```python
from build123d import *

# Parameters (mm, degrees)
ESQUISSE1_W                          = 6
ESQUISSE1_H                          = 3.2
EXTRUSION1_DEPTH                     = 22.64
ENL_V_MAT_EXTRU_1_DEPTH              = 0.5
ESQUISSE3_R                          = 0.25
R_P_TITION_LIN_AIRE1_COUNT           = 9
R_P_TITION_LIN_AIRE1_PITCH           = 2.54
R_P_TITION_LIN_AIRE1_COPY_1_SKETCH_R = 0.25
R_P_TITION_LIN_AIRE1_COPY_2_SKETCH_R = 0.25
R_P_TITION_LIN_AIRE1_COPY_3_SKETCH_R = 0.25
R_P_TITION_LIN_AIRE1_COPY_4_SKETCH_R = 0.25
R_P_TITION_LIN_AIRE1_COPY_5_SKETCH_R = 0.25
R_P_TITION_LIN_AIRE1_COPY_6_SKETCH_R = 0.25
R_P_TITION_LIN_AIRE1_COPY_7_SKETCH_R = 0.25
R_P_TITION_LIN_AIRE1_COPY_8_SKETCH_R = 0.25


with BuildPart() as part:
    # Esquisse1 → Extrusion1 (new body)
    with BuildSketch(Plane(origin=(0, 0, 0), x_dir=(0, 0, -1), z_dir=(1, 0, 0))):
        with Locations((0, 1.6)):
            Rectangle(ESQUISSE1_W, ESQUISSE1_H)
    extrude(amount=EXTRUSION1_DEPTH)

    # Esquisse2 → Enlèv. mat.-Extru.1 (cut)
    with BuildSketch(Plane(origin=(0, 3.2, 0), x_dir=(-1, 0, 0), z_dir=(0, 1, 0))):
        with BuildLine():
            Line((0, -1), (0, 1))
            ThreePointArc((0, 1), (-1, 0), (0, -1))
        make_face()
    extrude(amount=-ENL_V_MAT_EXTRU_1_DEPTH, mode=Mode.SUBTRACT)

    # Balayage1: sweep along a path in Esquisse5
    with BuildLine(Plane(origin=(1.16, 0, 0), x_dir=(0, 0, -1), z_dir=(1, 0, 0))) as balayage1_path:
        Line((-3, 1.6), (-3.65, 1.6))
        Line((-3.65, 1.6), (-3.65, -4))
    # Esquisse3 → Balayage1 (sweep)
    with BuildSketch(Plane.XY.offset(3)):
        with Locations((1.16, 1.6)):
            Circle(ESQUISSE3_R)
    balayage1 = sweep(path=balayage1_path.line, transition=Transition.RIGHT)

    # Symétrie1: Balayage1 across plane
    add(balayage1.mirror(Plane.XY))

    # Répétition linéaire1: Balayage1 ×9
    with Locations(*[(i * R_P_TITION_LIN_AIRE1_PITCH, 0, 0) for i in range(1, R_P_TITION_LIN_AIRE1_COUNT)]):
        add(balayage1)

    # Répétition linéaire1 copy 1: sweep along a path in Répétition linéaire1 copy 1 path
    with BuildLine(Plane(origin=(3.7, 0, 0), x_dir=(0, 0, 1), z_dir=(1, 0, 0))) as r_p_tition_lin_aire1_copy_1_path:
        Line((-3, -1.6), (-3.65, -1.6))
        Line((-3.65, -1.6), (-3.65, 4))
    # Répétition linéaire1 copy 1 sketch → Répétition linéaire1 copy 1 (sweep)
    with BuildSketch(Plane(origin=(2.54, 0, -3), x_dir=(1, 0, 0), z_dir=(0, 0, -1))):
        with Locations((1.16, -1.6)):
            Circle(R_P_TITION_LIN_AIRE1_COPY_1_SKETCH_R)
    sweep(path=r_p_tition_lin_aire1_copy_1_path.line, transition=Transition.RIGHT)

    # Répétition linéaire1 copy 2: sweep along a path in Répétition linéaire1 copy 2 path
    with BuildLine(Plane(origin=(6.24, 0, 0), x_dir=(0, 0, 1), z_dir=(1, 0, 0))) as r_p_tition_lin_aire1_copy_2_path:
        Line((-3, -1.6), (-3.65, -1.6))
        Line((-3.65, -1.6), (-3.65, 4))
    # Répétition linéaire1 copy 2 sketch → Répétition linéaire1 copy 2 (sweep)
    with BuildSketch(Plane(origin=(5.08, 0, -3), x_dir=(1, 0, 0), z_dir=(0, 0, -1))):
        with Locations((1.16, -1.6)):
            Circle(R_P_TITION_LIN_AIRE1_COPY_2_SKETCH_R)
    sweep(path=r_p_tition_lin_aire1_copy_2_path.line, transition=Transition.RIGHT)

    # Répétition linéaire1 copy 3: sweep along a path in Répétition linéaire1 copy 3 path
    with BuildLine(Plane(origin=(8.78, 0, 0), x_dir=(0, 0, 1), z_dir=(1, 0, 0))) as r_p_tition_lin_aire1_copy_3_path:
        Line((-3, -1.6), (-3.65, -1.6))
        Line((-3.65, -1.6), (-3.65, 4))
    # Répétition linéaire1 copy 3 sketch → Répétition linéaire1 copy 3 (sweep)
    with BuildSketch(Plane(origin=(7.62, 0, -3), x_dir=(1, 0, 0), z_dir=(0, 0, -1))):
        with Locations((1.16, -1.6)):
            Circle(R_P_TITION_LIN_AIRE1_COPY_3_SKETCH_R)
    sweep(path=r_p_tition_lin_aire1_copy_3_path.line, transition=Transition.RIGHT)

    # Répétition linéaire1 copy 4: sweep along a path in Répétition linéaire1 copy 4 path
    with BuildLine(Plane(origin=(11.32, 0, 0), x_dir=(0, 0, 1), z_dir=(1, 0, 0))) as r_p_tition_lin_aire1_copy_4_path:
        Line((-3, -1.6), (-3.65, -1.6))
        Line((-3.65, -1.6), (-3.65, 4))
    # Répétition linéaire1 copy 4 sketch → Répétition linéaire1 copy 4 (sweep)
    with BuildSketch(Plane(origin=(10.16, 0, -3), x_dir=(1, 0, 0), z_dir=(0, 0, -1))):
        with Locations((1.16, -1.6)):
            Circle(R_P_TITION_LIN_AIRE1_COPY_4_SKETCH_R)
    sweep(path=r_p_tition_lin_aire1_copy_4_path.line, transition=Transition.RIGHT)

    # Répétition linéaire1 copy 5: sweep along a path in Répétition linéaire1 copy 5 path
    with BuildLine(Plane(origin=(13.86, 0, 0), x_dir=(0, 0, 1), z_dir=(1, 0, 0))) as r_p_tition_lin_aire1_copy_5_path:
        Line((-3, -1.6), (-3.65, -1.6))
        Line((-3.65, -1.6), (-3.65, 4))
    # Répétition linéaire1 copy 5 sketch → Répétition linéaire1 copy 5 (sweep)
    with BuildSketch(Plane(origin=(12.7, 0, -3), x_dir=(1, 0, 0), z_dir=(0, 0, -1))):
        with Locations((1.16, -1.6)):
            Circle(R_P_TITION_LIN_AIRE1_COPY_5_SKETCH_R)
    sweep(path=r_p_tition_lin_aire1_copy_5_path.line, transition=Transition.RIGHT)

    # Répétition linéaire1 copy 6: sweep along a path in Répétition linéaire1 copy 6 path
    with BuildLine(Plane(origin=(16.4, 0, 0), x_dir=(0, 0, 1), z_dir=(1, 0, 0))) as r_p_tition_lin_aire1_copy_6_path:
        Line((-3, -1.6), (-3.65, -1.6))
        Line((-3.65, -1.6), (-3.65, 4))
    # Répétition linéaire1 copy 6 sketch → Répétition linéaire1 copy 6 (sweep)
    with BuildSketch(Plane(origin=(15.24, 0, -3), x_dir=(1, 0, 0), z_dir=(0, 0, -1))):
        with Locations((1.16, -1.6)):
            Circle(R_P_TITION_LIN_AIRE1_COPY_6_SKETCH_R)
    sweep(path=r_p_tition_lin_aire1_copy_6_path.line, transition=Transition.RIGHT)

    # Répétition linéaire1 copy 7: sweep along a path in Répétition linéaire1 copy 7 path
    with BuildLine(Plane(origin=(18.94, 0, 0), x_dir=(0, 0, 1), z_dir=(1, 0, 0))) as r_p_tition_lin_aire1_copy_7_path:
        Line((-3, -1.6), (-3.65, -1.6))
        Line((-3.65, -1.6), (-3.65, 4))
    # Répétition linéaire1 copy 7 sketch → Répétition linéaire1 copy 7 (sweep)
    with BuildSketch(Plane(origin=(17.78, 0, -3), x_dir=(1, 0, 0), z_dir=(0, 0, -1))):
        with Locations((1.16, -1.6)):
            Circle(R_P_TITION_LIN_AIRE1_COPY_7_SKETCH_R)
    sweep(path=r_p_tition_lin_aire1_copy_7_path.line, transition=Transition.RIGHT)

    # Répétition linéaire1 copy 8: sweep along a path in Répétition linéaire1 copy 8 path
    with BuildLine(Plane(origin=(21.48, 0, 0), x_dir=(0, 0, 1), z_dir=(1, 0, 0))) as r_p_tition_lin_aire1_copy_8_path:
        Line((-3, -1.6), (-3.65, -1.6))
        Line((-3.65, -1.6), (-3.65, 4))
    # Répétition linéaire1 copy 8 sketch → Répétition linéaire1 copy 8 (sweep)
    with BuildSketch(Plane(origin=(20.32, 0, -3), x_dir=(1, 0, 0), z_dir=(0, 0, -1))):
        with Locations((1.16, -1.6)):
            Circle(R_P_TITION_LIN_AIRE1_COPY_8_SKETCH_R)
    sweep(path=r_p_tition_lin_aire1_copy_8_path.line, transition=Transition.RIGHT)


solid = part.part
```
Verification items for the finished model (mm, model axes). A direction names the side the tool comes from. Round coordinates to 2 decimals unless told otherwise and drop trailing zeros. Order: outer loops, then holes, each group sorted by start corner. A loop starts at its lowest first (then second) coordinate and runs counter-clockwise, first axis right, second up. Notation, with made-up numbers: (67, 53.25) - (90, 53.25) arc R21 cw to (90, 57.25) - close; hole circle Ø2 at (62, 24.25). An arc over 180 degrees is marked (long way). Use CSV: the item, a comma, the result in double quotes.
(1) Access from +Z, -Z, +X, -X, +Y, -Y to the whole of each face (thin tool, end or side, straight path). Record for faces 4 (the face through (0, 2, 0)), 5 (the face through (11, 0, 0)).
Entries:
face 4,"+Z, -Z, -X, +Y, -Y"
face 5,"+X, -X, -Y"
(2) Section check A-A on y = -3.5. State how many separate pieces and enclosed holes the cut face has, and give its area (3 significant figures).
Entries:
separate pieces,"18"
enclosed holes,"0"
area,"3.53 mm^2"
(3) Mould release check, pull along Z, two halves, no side actions. Record for faces 1 (the face through (0.4, 2.7, 0)), 2 (the face through (1, 3, 0)), 3 (the face through (22.64, 2, 0)): released by +Z, released by -Z, zero draft, split by the parting line, or undercut.
Entries:
face 1,"undercut"
face 2,"undercut"
face 3,"zero draft"
(4) Gauge pin test, flat ends, axial feed: pin 1 Ø2 at (x, z) = (4.5, -2) entering from -Y; pin 2 Ø0.8 at (x, z) = (0.5, 0) entering from +Y; pin 3 Ø1 at (y, z) = (-3, -1) entering from -X. Record the tip position at first contact, or that the pin passes through.
Entries:
pin 1,"y = 0"
pin 2,"y = 2.7"
pin 3,"through"
(5) Section check C-C on x = 8.78. Record the boundary of the cut face in (y, z).
Entries:
outline,"(-4, -3.9) - (1.85, -3.9) - (1.85, -3) - (3.2, -3) - (3.2, 3) - (1.85, 3) - (1.85, 3.9) - (-4, 3.9) - (-4, 3.4) - (1.35, 3.4) - (1.35, 3) - (0, 3) - (0, -3) - (1.35, -3) - (1.35, -3.4) - (-4, -3.4) - close"
(6) Thickness scan on probe 1 along Z at (x, y) = (8.75, -3.5); probe 2 along Z at (x, y) = (13, 0.5); probe 3 along Y at (x, z) = (13.5, -0.25). Record the ranges inside material, lowest first. Write a range as from..to.
Entries:
probe 1,"-3.9..-3.4, 3.4..3.9"
probe 2,"-3..3"
probe 3,"0..3.2"
